```python
from build123d import *

# Parameters (mm, degrees)
F2_R     = 4.7917393222
F3_DEPTH = 25


# Not quite as in the source:
# - a fillet or chamfer that OpenCascade refuses, or shapes differently, is made with other operations: its cross-section is extruded or revolved along the edge and cut away or added


with BuildPart() as f1:
    # F0 (on Front) → F1 (revolve)
    with BuildSketch(Plane.XZ):
        Polygon((0, 12.9990037531), (0, 7.3299529031), (13.7201668695, 7.3299529031), (13.7201668695, 12.9990037531), (8.6628543213, 12.9990037531), (8.6628543213, 31.1359390616), (18.9999677241, 31.1359390616), (18.9999677241, 37.8080755472), (0, 37.8080755472), (0, 31.1359390616), (2.8364819009, 31.1359390616), (2.8364819009, 12.9990037531), align=None)
    revolve(axis=Axis((6.8600834347, 0, 0), (1, 0, 0)))

    # F2 (on face) → F3 (cut)
    with BuildSketch(Plane.YZ.offset(8.6628543213)):
        with Locations((-19.483606852, 6.3306076199)):
            Circle(F2_R)
        with Locations((0, 20.4862765968)):
            Circle(F2_R)
        with Locations((19.483606852, 6.3306076199)):
            Circle(F2_R)
        with Locations((12.041531258, -16.5737459183)):
            Circle(F2_R)
        with Locations((-12.041531258, -16.5737459183)):
            Circle(F2_R)
    extrude(amount=-F3_DEPTH, mode=Mode.SUBTRACT)

    # F4: fillet of radius 5 on 4 edges, made by hand

    # F4_s1 → F4_t2 (revolve, cut)
    with BuildSketch(Plane.XZ):
        with BuildLine():
            ThreePointArc((-0.0004, 32.8071098618), (1.4644660941, 36.3436094532), (5.0009656854, 37.8084755472))
            Line((5.0009656854, 37.8084755472), (5.0009656854, 38.3086121158))
            ThreePointArc((5.0009656854, 38.3086121158), (2.5004828427, 38.3082121158), (0, 38.3082121158))
            Line((0, 38.3082121158), (-0.5001365685, 37.8080755472))
            ThreePointArc((-0.5001365685, 37.8080755472), (-0.5001365685, 35.3075927045), (-0.5005365685, 32.8071098618))
            Line((-0.5005365685, 32.8071098618), (-0.0004, 32.8071098618))
        make_face()
    revolve(axis=Axis((0, 0, 0), (1, 0, 0)), mode=Mode.SUBTRACT)

    # F4_s3 → F4_t4 (revolve, cut)
    with BuildSketch(Plane.XZ):
        with BuildLine():
            ThreePointArc((13.9990020387, 37.8084755472), (17.53550163, 36.3436094532), (19.0003677241, 32.8071098618))
            Line((19.0003677241, 32.8071098618), (19.5005042926, 32.8071098618))
            ThreePointArc((19.5005042926, 32.8071098618), (19.5001042926, 35.3075927045), (19.5001042926, 37.8080755472))
            Line((19.5001042926, 37.8080755472), (18.9999677241, 38.3082121158))
            ThreePointArc((18.9999677241, 38.3082121158), (16.4994848814, 38.3082121158), (13.9990020387, 38.3086121158))
            Line((13.9990020387, 38.3086121158), (13.9990020387, 37.8084755472))
        make_face()
    revolve(axis=Axis((18.9999677241, 0, 0), (1, 0, 0)), mode=Mode.SUBTRACT)

    # F4_s5 → F4_t6 (revolve, cut)
    with BuildSketch(Plane.XZ):
        with BuildLine():
            ThreePointArc((-0.0004, 8.490714972), (0.7677695224, 11.1541167376), (2.8363087756, 12.9993643465))
            Line((2.8363087756, 12.9993643465), (2.6198430846, 13.450229284))
            ThreePointArc((2.6198430846, 13.450229284), (1.4181543878, 13.4991403216), (0, 13.4991403216))
            Line((0, 13.4991403216), (-0.5001365685, 12.9990037531))
            ThreePointArc((-0.5001365685, 12.9990037531), (-0.5001365685, 10.7448593625), (-0.5005365685, 8.490714972))
            Line((-0.5005365685, 8.490714972), (-0.0004, 8.490714972))
        make_face()
    revolve(axis=Axis((0, 0, 0), (1, 0, 0)), mode=Mode.SUBTRACT)

    # F4_s7 → F4_t8 (revolve, cut)
    with BuildSketch(Plane.XZ):
        with BuildLine():
            ThreePointArc((13.7205668695, 7.9980380676), (12.2557007754, 11.534537659), (8.719201184, 12.9994037531))
            Line((8.719201184, 12.9994037531), (8.719201184, 13.4995403216))
            ThreePointArc((8.719201184, 13.4995403216), (11.2196840267, 13.4991403216), (13.7201668695, 13.4991403216))
            Line((13.7201668695, 13.4991403216), (14.220303438, 12.9990037531))
            ThreePointArc((14.220303438, 12.9990037531), (14.220303438, 10.4985209104), (14.220703438, 7.9980380676))
            Line((14.220703438, 7.9980380676), (13.7205668695, 7.9980380676))
        make_face()
    revolve(axis=Axis((13.7201668695, 0, 0), (1, 0, 0)), mode=Mode.SUBTRACT)

    # F5: chamfer of 5 on 3 edges, made by hand

    # F5_s1 → F5_t2 (revolve, cut)
    with BuildSketch(Plane.XZ):
        Polygon((0, 12.3299529031), (5, 7.3299529031), (0, 7.3299529031), align=None)
    revolve(axis=Axis((0, 0, 0), (1, 0, 0)), mode=Mode.SUBTRACT)

    # F5_s3 → F5_t4 (revolve, cut)
    with BuildSketch(Plane.XZ):
        Polygon((8.7201668695, 7.3299529031), (13.7201668695, 12.3299529031), (13.7201668695, 7.3299529031), align=None)
    revolve(axis=Axis((13.7201668695, 0, 0), (1, 0, 0)), mode=Mode.SUBTRACT)


solid = f1.part
```
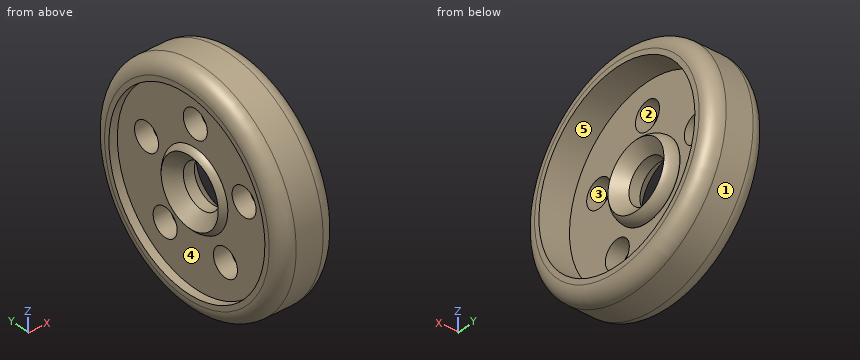
The listing builds one solid part. Answer for the finished solid, in the listing's coordinates (mm). Face numbers are marked on the shaded views. A direction names the side the tool comes from. Coordinates: 2 decimals unless noted, no trailing zeros. Write each loop counter-clockwise with the first axis right and the second up, starting at its lowest first coordinate (ties: lowest second). Pieces come first, ordered by that corner, then holes. Notation, with made-up numbers: (71.25, -36.5) -> (128.25, -36.5) arc R25 ccw to (128.25, -16.5) -> close; hole circle Ø5 at (-1.75, -3.5). An arc over 180 degrees is marked (long way). Write each question's results on one line, items separated by ' | '. Start each with the question number.
1) A cutting plane is placed at C-C (y = 0). Count the separate pieces of the cut face and the enclosed holes in it, then the cut area to 3 significant figures.
2) A tool of negligible diameter and unlimited length cuts with its end or side. For the marked faces 3, 4 and 5, from which of +Z, -Z, +X, -X, +Y, -Y can it reach the whole face along a straight path? Write none if from no direction.
3) A cutting plane is placed at B-B (x = 10.5). Determine the outline of the cut face in (y, z), then the cut area to 3 significant figures.
4) Flat-ended cylindrical pins translate along their axes: pin 1 Ø10 at (y, z) = (0.5, 7) entering from -X; pin 2 Ø5 at (x, z) = (9, -4.5) entering from +Y; pin 3 Ø6 at (x, y) = (11.5, -25) entering from +Z. Find the tip coordinate at first contact, or state that the pin passes through.
5) For a pull along Y with two mould halves and no side action, classify the marked faces 1 and 2 as +Y half, -Y half, draft (parallel to the pull), parting line (faces both ways), or undercut.
6) Straight lines are drawn through the part: probe 1 along Z at (x, y) = (7.25, 0); probe 2 along Y at (x, z) = (14.25, 0); probe 3 along Y at (x, z) = (2.1, 0). For each, find the intervals that lie inside material, in ascending order.
Values follow:
1) separate pieces: 3 | enclosed holes: 0 | area: 481 mm²
2) face 3: +X, -X | face 4: -X | face 5: +X
3) outline: circle Ø75.62 at (0, 0); circle Ø25.34 at (0, 0); hole circle Ø62.27 at (0, 0); hole circle Ø18.22 at (0, 0) | area: 1,690 mm²
4) pin 1: x = 0.93 | pin 2: y = 37.76 | pin 3: z = 30.75
5) face 1: parting line | face 2: undercut
6) probe 1: -37.81 to -7.33, 7.33 to 15.69, 25.28 to 37.81 | probe 2: -37.8 to -31.14, 31.14 to 37.8 | probe 3: -36.88 to -31.14, -12.56 to -10.23, 10.23 to 12.56, 31.14 to 36.88
